from build123d import *

# Parameters (mm, degrees)
SKETCH1_R           = 1.7
BOSS_EXTRUDE1_DEPTH = 5
SKETCH3_R           = 5
CUT_EXTRUDE1_DEPTH  = 4
CHAMFER1_SIZE       = 0.3


with BuildPart() as part:
    # Sketch1 → Boss-Extrude1 (new body)
    with BuildSketch(Plane.XY):
        with BuildLine():
            Line((-16.6225, -13.377), (-16.6225, 13.377))
            ThreePointArc((-16.6225, 13.377), (0, 29.9995), (16.6225, 13.377))
            Line((16.6225, 13.377), (16.6225, -13.377))
            ThreePointArc((16.6225, -13.377), (0, -29.9995), (-16.6225, -13.377))
        make_face()
        with Locations((0, -21)):
            Circle(SKETCH1_R, mode=Mode.SUBTRACT)
        with Locations((0, 21)):
            Circle(SKETCH1_R, mode=Mode.SUBTRACT)
    extrude(amount=BOSS_EXTRUDE1_DEPTH)

    # Sketch2 → Cut-Revolve1 (revolve, cut)
    with BuildSketch(Plane(origin=(0, 0, 0), x_dir=(0, 0, -1), z_dir=(1, 0, 0)), mode=Mode.PRIVATE) as cut_revolve1_sk:
        Polygon((0, -4.2), (-5, -4.2), (-5, -7.2), (-3.7, -5.9), (0, -5.9), align=None)
    revolve(cut_revolve1_sk.sketch.rotate(Axis((0, -4.2, 2.5), (0, 0, 1)), 180), axis=Axis((0, -4.2, 2.5), (0, 0, 1)), mode=Mode.SUBTRACT)

    # Sketch3 → Cut-Extrude1 (cut)
    with BuildSketch(Plane(origin=(0, 0, 0), x_dir=(-1, 0, 0), z_dir=(0, 0, -1))):
        with Locations((0, 21)):
            Circle(SKETCH3_R)
        with Locations((0, -21)):
            Circle(SKETCH3_R)
    extrude(amount=-CUT_EXTRUDE1_DEPTH, mode=Mode.SUBTRACT)

    # Chamfer1
    chamfer1_edges = [part.edges().sort_by_distance(p)[0] for p in [
        (5, 21, 0),
        (5, -21, 0),
    ]]
    chamfer(chamfer1_edges, length=CHAMFER1_SIZE)


solid = part.part
Geometry: final body of the model. Coordinates: model frame, mm. A direction names the side the tool comes from. Coordinates: 2 decimals unless noted, no trailing zeros. Order: outer loops, then holes, each group sorted by start corner. A loop starts at its lowest first (then second) coordinate and runs counter-clockwise, first axis right, second up. Notation, with made-up numbers: (54, 37) - (90, 37) arc R20 cw to (90, 68) - close; hole circle Ø11 at (31, 30). An arc over 180 degrees is marked (long way). Use one line per item in the form item = value.
1) Set-up query: faces 1 (the face through (0, 0, 5)), 2 (the face through (1.08, -25.88, 2.12)). Return all of +Z, -Z, +X, -X, +Y, -Y with unobstructed straight access to the full face (end or side cutting, diameter ignored); none if empty.
Solutions:
face_1 = +Z, +X, -X, +Y, -Y
face_2 = -Z
2) Pin query (flat end, axial travel): pin 1 (3 mm diameter, centred on x = -13, z = 2.5, fed in from +Y); pin 2 (3 mm diameter, centred on x = 1.5, y = -23, fed in from -Z); pin 3 (2.5 mm diameter, centred on x = 0, y = -21, fed in from +Z). Return the tip coordinate at first contact, or that it passes through.
Solutions:
pin_1 = 25.38
pin_2 = 4
pin_3 = through
3) Section B-B (y = -4.2). Return loops of the section in (x, z), then the cut area to 3 significant figures.
Solutions:
outline = (-16.62, 0) - (-1.7, 0) - (-1.7, 3.7) - (-3, 5) - (-16.62, 5) - close; (1.7, 0) - (16.62, 0) - (16.62, 5) - (3, 5) - (1.7, 3.7) - close
area = 148 mm^2
4) Mould query, pull axis Y, two halves, no side actions, for faces 3 (the face through (0, -30, 2)), 4 (the face through (-16.622, 0, 2)), 5 (the face through (0, 30, 2)), 6 (the face through (0.65, -2.63, 1.82)). Classes: +Y half, -Y half, draft (parallel to the pull), parting line (faces both ways), or undercut.
Solutions:
face_3 = -Y half
face_4 = draft
face_5 = +Y half
face_6 = undercut
5) Ray query, L1, parallel to Y at x = -2, z = 2.15; L2, parallel to Y at x = -1, z = 2.8; L3, parallel to X at y = -4.2, z = 2.45. Return the intervals inside material, ascending.
Solutions:
L1 = -29.88 to -25.58, -16.42 to 16.42, 25.58 to 29.88
L2 = -29.97 to -25.9, -16.1 to -5.57, -2.83 to 16.1, 25.9 to 29.97
L3 = -16.62 to -1.7, 1.7 to 16.62
6) Section C-C (z = 1.75). Return loops of the section in (x, y) (1 decimal).
Solutions:
outline = (-16.6, -13.4) arc R16.6 ccw to (16.6, -13.4) - (16.6, 13.4) arc R16.6 ccw to (-16.6, 13.4) - close; hole circle Ø10 at (0, -21); hole circle Ø10 at (0, 21); hole circle Ø3.4 at (0, -4.2)
7) Section A-A (x = 0). State how many separate pieces and enclosed holes the cut face has, then the cut area to 3 significant figures.
Solutions:
separate_pieces = 4
enclosed_holes = 0
area = 194 mm^2
8) Section D-D (y = -21). Return loops of the section in (x, z), then the cut area to 3 significant figures.
Solutions:
outline = (-14.77, 0) - (-5.3, 0) - (-5, 0.3) - (-5, 4) - (-1.7, 4) - (-1.7, 5) - (-14.77, 5) - close; (1.7, 4) - (5, 4) - (5, 0.3) - (5.3, 0) - (14.77, 0) - (14.77, 5) - (1.7, 5) - close
area = 104 mm^2
